For this review, take the finished solid that the model builds, in its own axes (mm). A direction names the side the tool comes from. Round coordinates to 2 decimals unless told otherwise and drop trailing zeros. Write each loop counter-clockwise with the first axis right and the second up, starting at its lowest first coordinate (ties: lowest second). Pieces come first, ordered by that corner, then holes.
from build123d import *

# Parameters (mm, degrees)
BOSS_EXTRUDE1_DEPTH  = 6.35
FILLET1_R            = 3
M3_CLEARANCE_HOLE1_D = 3.4


with BuildPart() as part:
    # Sketch2 → Boss-Extrude1 (new body)
    with BuildSketch(Plane.XY):
        with BuildLine():
            Line((-14, 39.75), (-14, 9))
            ThreePointArc((-14, 9), (-13.621112393, 6.728245023), (-12.525465522, 4.702415705))
            Line((-12.525465522, 4.702415705), (-5.525465522, -4.297584295))
            ThreePointArc((-5.525465522, -4.297584295), (-3.075460123, -6.288206822), (0, -7))
            Line((0, -7), (41.5, -7))
            ThreePointArc((41.5, -7), (48.5, 0), (41.5, 7))
            Line((41.5, 7), (0, 7))
            Line((0, 7), (0, 39.75))
            ThreePointArc((0, 39.75), (-7, 46.75), (-14, 39.75))
        make_face()
    extrude(amount=BOSS_EXTRUDE1_DEPTH)

    # Fillet1
    fillet1_edges = [part.edges().sort_by_distance(p)[0] for p in [
        (0, 7, 3.175),
    ]]
    fillet(fillet1_edges, radius=FILLET1_R)

    # M3 Clearance Hole1 (through all)
    with Locations(Plane.XY.offset(6.35)):
        with Locations((-7, 39.75), (-7, 9), (0, 0), (41.5, 0)):
            Hole(M3_CLEARANCE_HOLE1_D / 2)


solid = part.part
(1) For pin 1 Ø5.5 at (x, y) = (-7, 9) entering from -Z; pin 2 Ø3 at (y, z) = (32, 4.5) entering from +X; pin 3 Ø2 at (x, z) = (23.5, 4.5) entering from +Y, all flat-tipped, find the tip position at first contact; note any pin that passes through.
Geometry check:
pin 1: stops at z = 0
pin 2: stops at x = 0
pin 3: stops at y = 7
(2) We need section B-B, the plane x = -7. Give the boundary of the cut face in (y, z).
Geometry check:
outline: (-2.4, 0) - (7.3, 0) - (7.3, 6.35) - (-2.4, 6.35) - close; (10.7, 0) - (38.05, 0) - (38.05, 6.35) - (10.7, 6.35) - close; (41.45, 0) - (46.75, 0) - (46.75, 6.35) - (41.45, 6.35) - close
(3) For line 1 along Y through (x, z) = (-7, 2); line 2 along X through (y, z) = (-1, 5.5); line 3 along X through (y, z) = (20.5, 5.5), list the stretches that pass through material, from the lowest coordinate up.
Geometry check:
line 1: y = -2.4 to 7.3, 10.7 to 38.05, 41.45 to 46.75
line 2: x = -8.09 to -1.37, 1.37 to 40.13, 42.87 to 48.43
line 3: x = -14 to 0
(4) We need section D-D, the plane y = 29.5. Give the boundary of the cut face in (x, z).
Geometry check:
outline: (-14, 0) - (0, 0) - (0, 6.35) - (-14, 6.35) - close
(5) Mouldability with a two-part tool opening along X and no side actions: class faces 1 (the face through (-6.63, 7.34, 3.13)), 2 (the face through (-6.85, 46.75, 3.13)), 3 (the face through (23, 7, 3)) as pulls with the +X half, pulls with the -X half, needs draft (parallel to the pull), parting line crosses it, or undercut.
Geometry check:
face 1: undercut
face 2: parting line crosses it
face 3: needs draft
(6) We need section C-C, the plane y = 0. Give the boundary of the cut face in (x, z), and give its area (3 significant figures).
Geometry check:
outline: (-8.87, 0) - (-1.7, 0) - (-1.7, 6.35) - (-8.87, 6.35) - close; (1.7, 0) - (39.8, 0) - (39.8, 6.35) - (1.7, 6.35) - close; (43.2, 0) - (48.5, 0) - (48.5, 6.35) - (43.2, 6.35) - close
area: 321 mm2
(7) We need section A-A, the plane z = 4. Give the boundary of the cut face in (x, y).
Geometry check:
outline: (-14, 9) arc R7 ccw to (-12.53, 4.7) - (-5.53, -4.3) arc R7 ccw to (0, -7) - (41.5, -7) arc R7 ccw to (41.5, 7) - (3, 7) arc R3 cw to (0, 10) - (0, 39.75) arc R7 ccw to (-14, 39.75) - close; hole circle Ø3.4 at (-7, 9); hole circle Ø3.4 at (-7, 39.75); hole circle Ø3.4 at (0, 0); hole circle Ø3.4 at (41.5, 0)
(8) For faces 4 (the face through (-9.1, 0.3, 3.1)), 5 (the face through (0, 25, 3)), list the 3-axis set-ups (+Z, -Z, +X, -X, +Y, -Y) from which the entire face can be reached by the end or side of a thin tool; tool diameter is ignored.
Geometry check:
face 4: +Z, -Z, -X, -Y
face 5: +Z, -Z, +X, +Y
